Autodesk Inventor part; units mm, degrees
ref_plane "YZ Plane" through (0, 0, 0) normal (1, 0, 0) x (0, 1, 0)
ref_plane "XZ Plane" through (0, 0, 0) normal (0, 1, 0) x (-1, 0, 0)
ref_plane "XY Plane" through (0, 0, 0) normal (0, 0, 1) x (1, 0, 0)
sketch "Sketch1" plane through (0, 0, 0) normal (0, 0, 1) x (1, 0, 0)
  line L0 (15.875, 15.875) -> (-15.875, 15.875)
  line L1 (-15.875, 15.875) -> (-15.875, -15.875)
  line L2 (-15.875, -15.875) -> (15.875, -15.875)
  line L3 (15.875, -15.875) -> (15.875, 15.875)
  line L4 (15.875, 15.875) -> (-15.875, -15.875) construction
  line L5 (-15.875, 15.875) -> (15.875, -15.875) construction
  point P0 (0, 0)
  dimension "d0" = 31.75
  dimension "d1" = 31.75
extrude "Extrusion1" add sketch "Sketch1" along normal blind 1.27
sketch "Sketch2" plane through (0, 0, 1.27) normal (0, 0, 1) x (1, 0, 0)
  line L0 (-10.16, 10.16) -> (10.16, 10.16)
  line L1 (10.16, 10.16) -> (10.16, -10.16)
  line L2 (10.16, -10.16) -> (-10.16, -10.16)
  line L3 (-10.16, -10.16) -> (-10.16, 10.16)
  line L4 (15.875, 15.875) -> (-15.875, 15.875)
  line L5 (15.875, -15.875) -> (15.875, 15.875)
  line L6 (-15.875, -15.875) -> (15.875, -15.875)
  line L7 (-15.875, 15.875) -> (-15.875, -15.875)
  point P0 (0, 0)
  dimension "d4" = 5.715
  dimension "d5" = 5.715
  dimension "d6" = 5.715
  dimension "d7" = 5.715
extrude "Extrusion2" add sketch "Sketch2" along normal blind 1.27 contours L0 L1 L2 L3
sketch "Sketch3" plane through (0, 0, 2.54) normal (0, 0, 1) x (1, 0, 0)
  line L0 (-8.255, 8.255) -> (8.255, 8.255)
  line L1 (8.255, 8.255) -> (8.255, 4.953)
  line L2 (8.255, 4.953) -> (-8.255, 4.953)
  line L3 (-8.255, 4.953) -> (-8.255, 8.255)
  line L4 (10.16, -10.16) -> (10.16, 10.16)
  line L5 (-10.16, 10.16) -> (-10.16, -10.16)
  line L6 (10.16, 10.16) -> (-10.16, 10.16)
  line L7 (-8.255, -8.255) -> (8.255, -8.255)
  line L8 (8.255, -8.255) -> (8.255, -4.953)
  line L9 (8.255, -4.953) -> (-8.255, -4.953)
  line L10 (-8.255, -4.953) -> (-8.255, -8.255)
  line L11 (-10.16, -10.16) -> (10.16, -10.16)
  point P0 (0, 0)
  dimension "d10" = 1.905
  dimension "d11" = 1.905
  dimension "d12" = 1.905
  dimension "d14" = 1.905
  dimension "d15" = 1.905
  dimension "d16" = 1.905
  dimension "d39" = 9.906
  dimension "d40" = 3.302
  dimension "d41" = 3.302
extrude "Extrusion3" add sketch "Sketch3" along normal blind 19.05 contours L0 L1 L2 L3 | L10 L9 L8 L7
sketch "Sketch4" plane through (-8.255, -8.255, 2.54) normal (0, -1, 0) x (1, 0, 0)
  circle A0 centre (10.16, 11.43) radius 3.175
  line L0 (0, 19.05) -> (16.51, 19.05)
  line L1 (0, 0) -> (0, 19.05)
  point P0 (8.255, -2.54)
  dimension "d20" = 6.35
  dimension "d21" = 7.62
  dimension "d44" = 10.16
extrude "Extrusion4" cut sketch "Sketch4" against normal blind 127
sketch "Sketch5" plane through (0, 0, 1.27) normal (0, 0, 1) x (1, 0, 0)
  circle A0 centre (-12.065, 12.065) radius 2.5797
  line L0 (-15.875, -15.875) -> (15.875, -15.875)
  line L1 (15.875, -15.875) -> (15.875, 15.875)
  circle A1 centre (12.065, 12.065) radius 2.5797
  line L2 (15.875, 15.875) -> (-15.875, 15.875)
  line L3 (-15.875, 15.875) -> (-15.875, -15.875)
  circle A2 centre (-12.065, -12.065) radius 2.5797
  circle A3 centre (12.065, -12.065) radius 2.5797
  point P0 (0, 0)
  dimension "d24" = 5.1594
  dimension "d28" = 5.1594
  dimension "d29" = 3.81
  dimension "d30" = 3.81
  dimension "d31" = 3.81
  dimension "d32" = 3.81
  dimension "d33" = 5.1594
  dimension "d34" = 3.81
  dimension "d35" = 3.81
  dimension "d36" = 5.1594
  dimension "d37" = 3.81
  dimension "d38" = 3.81
extrude "Extrusion5" cut sketch "Sketch5" against normal blind 12.7 contours A0 | A1 | A2 | A3
sketch "Sketch6" plane through (-8.255, -8.255, 2.54) normal (0, -1, 0) x (1, 0, 0)
  line L0 (0, 0) -> (0, 19.05)
  line L1 (0, 19.05) -> (16.51, 19.05)
  line L2 (0, 6.5528) -> (5.4184, 6.5528)
  line L3 (5.4184, 6.5528) -> (5.4184, 19.05)
  line L4 (5.4184, 19.05) -> (0, 19.05)
  line L5 (0, 19.05) -> (0, 6.5528)
  point P0 (8.255, -2.54)
extrude "Extrusion6" cut sketch "Sketch6" against normal blind 101.6
equation "\"d5\" = d4"
equation "\"d6\" = d4"
equation "\"d7\" = d4"
equation "\"d11\" = d10"
equation "\"d12\" = d10"
equation "\"d14\" = d10"
equation "\"d15\" = d10"
equation "\"d16\" = d10"
equation "\"d28\" = d24"
equation "\"d30\" = d29"
equation "\"d31\" = d29"
equation "\"d32\" = d29"
equation "\"d33\" = d24"
equation "\"d34\" = d29"
equation "\"d35\" = d29"
equation "\"d36\" = d24"
equation "\"d37\" = d29"
equation "\"d38\" = d29"
properties part number "pneumatics back holder"
Model file for the job. Use its own axes, mm. A direction names the side the tool comes from. Give positions to 0.01 mm unless a question says otherwise; leave off trailing zeros. Loops run counter-clockwise (first coordinate to the right, second up) from the corner with the lowest first, then second, coordinate; pieces in that order, holes last. Notation, with made-up numbers: (66.5, 20.25) -> (72.5, 20.25) arc R27 cw to (72.5, 44.25) -> close; hole circle Ø1 at (32.5, -9.5). An arc over 180 degrees is marked (long way). Write each question's results on one line, items separated by ' | '.
(1) Cut at A-A on z = 5.5. List the corners of the cut face in (x, y) (3 decimals), and give its area (3 significant figures).
Geometry results:
outline: (-8.255, -8.255) -> (8.255, -8.255) -> (8.255, -4.953) -> (-8.255, -4.953) -> close; (-8.255, 4.953) -> (8.255, 4.953) -> (8.255, 8.255) -> (-8.255, 8.255) -> close | area: 109 mm²
(2) Flat gauge pins, fed straight in: pin 1 Ø2 at (x, z) = (9, 7.5) entering from +Y (3 decimals); pin 2 Ø1.7 at (y, z) = (-7, 12.5) entering from +X (3 decimals); pin 3 Ø10 at (y, z) = (7, 18) entering from -X. Where does each tip first touch, or does it go through?
Geometry results:
pin 1: stops at y = 8.255 | pin 2: stops at x = 8.255 | pin 3: stops at x = -2.84
(3) Probe line 1 along Y through (x, z) = (-8, 7) (3 decimals); line 2 along Z through (x, y) = (2.5, -2.5); line 3 along Z through (x, y) = (14, 0). List the from-to ranges inside material, lowest first.
Geometry results:
line 1: y = -8.255 to -4.953, 4.953 to 8.255 | line 2: z = 0 to 2.54 | line 3: z = 0 to 1.27
(4) Cut at C-C on x = 9. List the corners of the cut face in (y, z) (3 decimals), and give its area (3 significant figures).
Geometry results:
outline: (-15.875, 0) -> (15.875, 0) -> (15.875, 1.27) -> (10.16, 1.27) -> (10.16, 2.54) -> (-10.16, 2.54) -> (-10.16, 1.27) -> (-15.875, 1.27) -> close | area: 66.1 mm²
(5) Tool access for faces 1 (the flat face through (2, -4.953, 10)), 2 (the flat face through (-6, 7, 9.093)), 3 (the flat face through (8.255, 7, 12)): list every direction of +Z, -Z, +X, -X, +Y, -Y with a clear straight run to the whole face (end or side of a thin tool).
Geometry results:
face 1: +Z, +X, -X | face 2: +Z, -X, +Y, -Y | face 3: +Z, +X, +Y, -Y
(6) Cut at D-D on z = 13.97. List the corners of the cut face in (x, y) (3 decimals).
Geometry results:
outline: (-2.837, -8.255) -> (-1.27, -8.255) -> (-1.27, -4.953) -> (-2.837, -4.953) -> close; (-2.837, 4.953) -> (-1.27, 4.953) -> (-1.27, 8.255) -> (-2.837, 8.255) -> close; (5.08, -8.255) -> (8.255, -8.255) -> (8.255, -4.953) -> (5.08, -4.953) -> close; (5.08, 4.953) -> (8.255, 4.953) -> (8.255, 8.255) -> (5.08, 8.255) -> close
(7) Pull direction Y, two halves, no side cores. Call faces 4 (the flat face through (3, -7, 21.59)), 5 (the flat face through (2, 8.255, 10)), 6 (the cylindrical face through (-9.604, 12.84, 0.644)): released by +Y, released by -Y, zero draft, split by the parting line, or undercut.
Geometry results:
face 4: zero draft | face 5: released by +Y | face 6: undercut
(8) Cut at B-B on y = 6. List the corners of the cut face in (x, z) (3 decimals), and give its area (3 significant figures).
Geometry results:
outline: (-15.875, 0) -> (15.875, 0) -> (15.875, 1.27) -> (10.16, 1.27) -> (10.16, 2.54) -> (8.255, 2.54) -> (8.255, 21.59) -> (-2.837, 21.59) -> (-2.837, 9.093) -> (-8.255, 9.093) -> (-8.255, 2.54) -> (-10.16, 2.54) -> (-10.16, 1.27) -> (-15.875, 1.27) -> close; hole circle Ø6.35 at (1.905, 13.97) | area: 281 mm²
